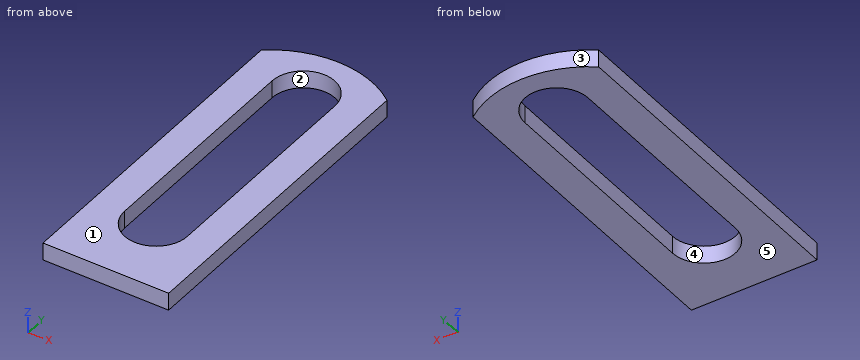
from build123d import *

# Parameters (mm, degrees)
BOSS_EXTRUDE1_DEPTH = 2.8


with BuildPart() as part:
    # Sketch1 → Boss-Extrude1 (new body)
    with BuildSketch(Plane.XY.offset(2.8)):
        with BuildLine():
            Line((0, 52.179630025), (0, 0))
            Line((0, 0), (20.2, 0))
            Line((20.2, 0), (20.2, 52.179630025))
            ThreePointArc((20.2, 52.179630025), (10.1, 55.643160629), (0, 52.179630025))
        make_face()
        with BuildLine():
            Line((15.15, 47.222342094), (15.15, 12))
            ThreePointArc((15.15, 12), (10.1, 6.95), (5.05, 12))
            Line((5.05, 12), (5.05, 47.222342094))
            ThreePointArc((5.05, 47.222342094), (10.1, 52.272342094), (15.15, 47.222342094))
        make_face(mode=Mode.SUBTRACT)
    extrude(amount=-BOSS_EXTRUDE1_DEPTH)


solid = part.part
Work out the finished part from the listing and answer in its coordinate system (mm). Face numbers are marked on the shaded views. A direction names the side the tool comes from. Give positions to 0.01 mm unless a question says otherwise; leave off trailing zeros. Order: outer loops, then holes, each group sorted by start corner. A loop starts at its lowest first (then second) coordinate and runs counter-clockwise, first axis right, second up. Notation, with made-up numbers: (61.5, -38) -> (88.5, -38) arc R12 ccw to (88.5, -24) -> close; hole circle Ø8 at (-24, -10.75). An arc over 180 degrees is marked (long way). Answer as a JSON object with one key per item and string values. Group by question number.
1. Section C-C on z = 0.85 is taken. Determine the outline of the cut face in (x, y), plus the area to 3 significant figures.
2. Consider line 1 along X through (y, z) = (19.5, 0.85); line 2 along Y through (x, z) = (9.75, 0.7); line 3 along Y through (x, z) = (12.5, 0.45). Determine where each line is inside the solid, lowest interval first. Write a range as [from, to].
3. Section D-D on x = 18 is taken. Determine the outline of the cut face in (y, z), plus the area to 3 significant figures.
4. A tool of negligible diameter and unlimited length cuts with its end or side. For the marked faces 1 and 2, from which of +Z, -Z, +X, -X, +Y, -Y can it reach the whole face along a straight path? Write none if from no direction.
5. The mould has two halves that part along X. Classify the marked faces 3, 4 and 5: released by +X, released by -X, zero draft, split by the parting line, or undercut.
6. A flat-ended cylindrical pin translates along its axis: pin 1 Ø1 at (x, z) = (12.5, 2) entering from -Y. Find the tip coordinate at first contact, or state that the pin passes through.
7. Section B-B on y = 20 is taken. Determine the outline of the cut face in (x, z), plus the area to 3 significant figures.
8. Section A-A on x = 10.1 is taken. Determine the outline of the cut face in (y, z).
Result sheet:
{
 "1": {"outline": "(0, 0) -> (20.2, 0) -> (20.2, 52.18) arc R16.46 ccw to (0, 52.18) -> close; hole (5.05, 12) arc R5.05 ccw to (15.15, 12) -> (15.15, 47.22) arc R5.05 ccw to (5.05, 47.22) -> close", "area": "666 mm^2"},
 "2": {"line 1": "x = [0, 5.05], [15.15, 20.2]", "line 2": "y = [0, 6.96], [52.26, 55.64]", "line 3": "y = [0, 7.56], [51.67, 55.47]"},
 "3": {"outline": "(0, 0) -> (53.62, 0) -> (53.62, 2.8) -> (0, 2.8) -> close", "area": "150 mm^2"},
 "4": {"face 1": "+Z, +X, -X, +Y, -Y", "face 2": "+Z, -Z"},
 "5": {"face 3": "split by the parting line", "face 4": "undercut", "face 5": "zero draft"},
 "6": {"pin 1": "stops at y = 0"},
 "7": {"outline": "(0, 0) -> (5.05, 0) -> (5.05, 2.8) -> (0, 2.8) -> close; (15.15, 0) -> (20.2, 0) -> (20.2, 2.8) -> (15.15, 2.8) -> close", "area": "28.3 mm^2"},
 "8": {"outline": "(0, 0) -> (6.95, 0) -> (6.95, 2.8) -> (0, 2.8) -> close; (52.27, 0) -> (55.64, 0) -> (55.64, 2.8) -> (52.27, 2.8) -> close"}
}
